Could you check a few things on this model? Use its own coordinates, in mm. Face numbers are marked on the shaded views. Round coordinates to 2 decimals unless told otherwise and drop trailing zeros. Loops run counter-clockwise (first coordinate to the right, second up) from the corner with the lowest first, then second, coordinate; pieces in that order, holes last. Notation, with made-up numbers: (84, 44) - (104, 44) arc R17 ccw to (104, 48) - close; hole circle Ø9 at (-29.75, 80). An arc over 180 degrees is marked (long way). Use one line per item in the form item = value.
```python
from build123d import *

# Parameters (mm, degrees)
F0_W     = 450
F0_H     = 450
F1_DEPTH = 950
F2_W     = 329.7586178293
F2_H     = 475
F2_W_2   = 50
F2_H_2   = 50
F3_DEPTH = 450.001
F4_W     = 380
F4_H     = 490
F5_DEPTH = 450.001
F6_W     = 382.2745978832
F6_H     = 50
F6_H_2   = 252.9310692156
F7_DEPTH = 446.9187719453


with BuildPart() as f1:
    # F0 (on Top) → F1 (new body)
    with BuildSketch(Plane.XY):
        Rectangle(F0_W, F0_H)
    extrude(amount=F1_DEPTH)

    # F2 (on face) → F3 (cut, through all)
    with BuildSketch(Plane.XZ.offset(225)):
        Polygon((-225, 950), (-225, 525), (139.7586178293, 525), (189.7586178293, 950), align=None)
        with Locations((-25.1206910853, 237.5)):
            Rectangle(F2_W, F2_H)
        Polygon((225, 950), (175, 525), (225, 525), align=None)
        with Locations((200, 500)):
            Rectangle(F2_W_2, F2_H_2)
        with Locations((200, 237.5)):
            Rectangle(F2_W_2, F2_H)
    extrude(amount=-F3_DEPTH, mode=Mode.SUBTRACT)

    # F4 (on face) → F5 (cut, through all)
    with BuildSketch(Plane(origin=(-225, 0, 0), x_dir=(0, -1, 0), z_dir=(-1, 0, 0))):
        with Locations((0, 245)):
            Rectangle(F4_W, F4_H)
    extrude(amount=-F5_DEPTH, mode=Mode.SUBTRACT)

    # F6 (on face) → F7 (cut, through all)
    with BuildSketch(Plane(origin=(111.6894197952, 0, -13.1399317406), x_dir=(0, 1, 0), z_dir=(0.9931506043, 0, -0.1168412476))):
        with Locations((-0.9801834822, 869.7823548094)):
            Rectangle(F6_W, F6_H)
        with Locations((-0.9801834822, 668.3168202016)):
            Rectangle(F6_W, F6_H_2)
    extrude(amount=-F7_DEPTH, mode=Mode.SUBTRACT)


solid = f1.part
```
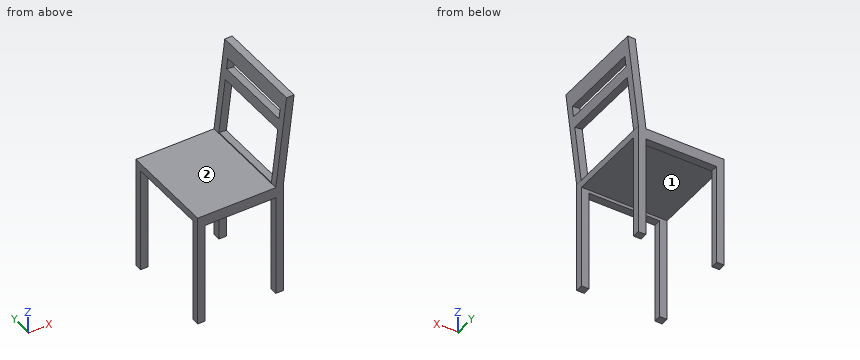
1. For P1, Ø17.5, axis at x = -67, y = -207, coming from the -Z side; P2, Ø3, axis at x = -150, y = 39, coming from the -Z side; P3, Ø17.5, axis at y = -208.5, z = 132.5, coming from the +X side, each with a flat end and sliding along its axis, tell me the tip position at first contact or that it passes through.
Solution:
P1 = 475
P2 = 490
P3 = 175
2. If we section it at C-C, the plane z = 692: Write out the boundary of the cut face in (x, y), plus the area to 3 significant figures.
Solution:
outline = (159.41, -225) - (194.65, -225) - (194.65, -192.12) - (159.41, -192.12) - close; (159.41, 190.16) - (194.65, 190.16) - (194.65, 225) - (159.41, 225) - close
area = 2,390 mm^2
3. Please list where these lines run through material, in increasing order: line 1 along Y through (x, z) = (-66.5, 481.5); line 2 along X through (y, z) = (-200, 198.5); line 3 along Z through (x, y) = (126.5, 137.5).
Solution:
line_1 = -225 to -190, 190 to 225
line_2 = -225 to -190, 139.76 to 175
line_3 = 490 to 525
4. If we section it at D-D, the plane x = 21.5: Write out the boundary of the cut face in (y, z).
Solution:
outline = (-225, 475) - (-190, 475) - (-190, 490) - (190, 490) - (190, 475) - (225, 475) - (225, 525) - (-225, 525) - close
5. If we section it at A-A, the plane z = 68.5: Write out the boundary of the cut face in (x, y), plus the area to 3 significant figures.
Solution:
outline = (-225, -225) - (-190, -225) - (-190, -190) - (-225, -190) - close; (-225, 190) - (-190, 190) - (-190, 225) - (-225, 225) - close; (139.76, -225) - (175, -225) - (175, -190) - (139.76, -190) - close; (139.76, 190) - (175, 190) - (175, 225) - (139.76, 225) - close
area = 4,920 mm^2
6. If we section it at B-B, the plane y = -140.5: Write out the boundary of the cut face in (x, z).
Solution:
outline = (-225, 490) - (175, 490) - (175, 525) - (140.24, 529.09) - (139.76, 525) - (-225, 525) - close; (169.79, 780.29) - (204.55, 776.2) - (210.39, 825.86) - (175.63, 829.95) - close; (181.48, 879.6) - (216.24, 875.51) - (225, 950) - (189.76, 950) - close
7. We'd pull the mould along Y, two halves only. Please class the marked faces 1 and 2: +Y half, -Y half, draft (parallel to the pull), parting line (faces both ways), or undercut.
Solution:
face_1 = undercut
face_2 = draft
